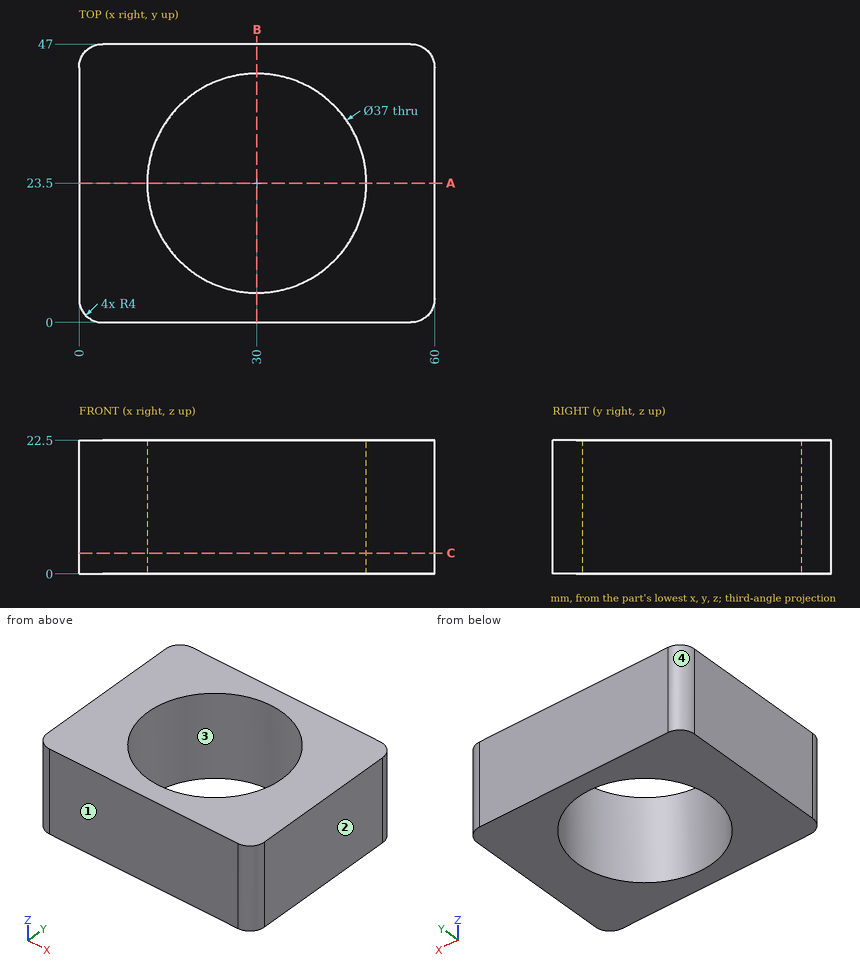
The figure shows three views and two pictorial views of one solid part (mm, origin at its lowest corner). Answer the questions. Coordinates: 2 decimals unless noted, no trailing zeros. Loops run counter-clockwise (first coordinate to the right, second up) from the corner with the lowest first, then second, coordinate; pieces in that order, holes last. Notation, with made-up numbers: (27, 18) - (65, 18) arc R11 ccw to (65, 29) - close; hole circle Ø2 at (22, 19.5). An arc over 180 degrees is marked (long way). Use a Markdown table: item, result. Add a question column.
1) The mould has two halves that part along X. Classify the marked faces 1, 2, 3 and 4: released by +X, released by -X, zero draft, split by the parting line, or undercut.
2) The part is cut by section B-B, the plane x = 30. Give the vertices of the cut face in (y, z).
3) Find the intervals of material crossed by line 1 (Y direction, x = 30, z = 10); line 2 (X direction, y = 17.5, z = 3.25); line 3 (X direction, y = 7, z = 7.25), in increasing order.
4) The part is cut by section C-C, the plane z = 3.5. Give the vertices of the cut face in (x, y).
5) The part is cut by section A-A, the plane y = 23.5. Give the vertices of the cut face in (x, z), and give its area (4 significant figures).
Here are the results:
| question | item | result |
|---|---|---|
| 1 | face 1 | zero draft |
| 1 | face 2 | released by +X |
| 1 | face 3 | undercut |
| 1 | face 4 | released by -X |
| 2 | outline | (0, 0) - (5, 0) - (5, 22.5) - (0, 22.5) - close; (42, 0) - (47, 0) - (47, 22.5) - (42, 22.5) - close |
| 3 | line 1 | y = 0 to 5, 42 to 47 |
| 3 | line 2 | x = 0 to 12.5, 47.5 to 60 |
| 3 | line 3 | x = 0 to 21.63, 38.37 to 60 |
| 4 | outline | (0, 4) arc R4 ccw to (4, 0) - (56, 0) arc R4 ccw to (60, 4) - (60, 43) arc R4 ccw to (56, 47) - (4, 47) arc R4 ccw to (0, 43) - close; hole circle Ø37 at (30, 23.5) |
| 5 | outline | (0, 0) - (11.5, 0) - (11.5, 22.5) - (0, 22.5) - close; (48.5, 0) - (60, 0) - (60, 22.5) - (48.5, 22.5) - close |
| 5 | area | 517.5 mm^2 |
